Check sheet for the modelled part. Datum: model origin and axes. Units: mm. A direction names the side the tool comes from. Round coordinates to 2 decimals unless told otherwise and drop trailing zeros. Order: outer loops, then holes, each group sorted by start corner. A loop starts at its lowest first (then second) coordinate and runs counter-clockwise, first axis right, second up. Notation, with made-up numbers: (40.25, -4) -> (53.25, -4) arc R22 cw to (53.25, 4) -> close; hole circle Ø2 at (-14.5, 58.25). An arc over 180 degrees is marked (long way). Answer in a Markdown table with one row per item. Add a question column.
1. Sectioned sample at B-B, the plane z = 0. Record the boundary of the cut face in (x, y).
2. Sectioned sample at A-A, the plane x = 0. Record the boundary of the cut face in (y, z), then the cut area to 3 significant figures.
3. Depth check by flat-ended pin: P1, Ø1, axis at x = 5.5, y = 13, coming from the -Z side; P2, Ø1.5, axis at x = 2.5, y = -65.5, coming from the +Z side; P3, Ø1.5, axis at x = -5.5, z = 5.5, coming from the -Y side. Enter the tip coordinate at first touch or a pass-through.
4. Access from +Z, -Z, +X, -X, +Y, -Y to the whole of each face (thin tool, end or side, straight path). Record for faces 1 (the flat face through (-6, -24.5, -3)), 2 (the cylindrical face through (-5.158, -65.845, 3.955)), 3 (the flat face through (0, -105, 0)).
5. Material ranges on L1, parallel to Y at x = 0, z = -7; L2, parallel to Z at x = 3, y = 35; L3, parallel to Z at x = 2.25, y = -76.5, recorded low to high. Write a range as from..to.
6. Sectioned sample at C-C, the plane y = 29.5. Record the boundary of the cut face in (x, z).
Solid Edge part; units mm, degrees
sketch "Sketch1" plane through (0, 0, 0) normal (0, -1, 0) x (1, 0, 0)
  circle A0 centre (0, 0) radius 6.5
extrude "Protrusion1" add sketch "Sketch1" along normal mid plane 210
sketch "Sketch2" plane through (0, -28.5, 0) normal (0, -1, 0) x (0, 0, -1)
  circle A0 centre (0, 0) radius 9
extrude "ExtrudedProtrusion_2" add sketch "Sketch2" against normal blind 4
chamfer "Chamfer_1" distance 0.75 angle 45 1 edges at (-6.5, -105, 0)
properties part number "SMV-102-4" material "STEEL, 4140"
Answer key:
| question | item | result |
|---|---|---|
| 1 | outline | (-9, -28.5) -> (-6.5, -28.5) -> (-6.5, -104.25) -> (-5.75, -105) -> (5.75, -105) -> (6.5, -104.25) -> (6.5, -28.5) -> (9, -28.5) -> (9, -24.5) -> (6.5, -24.5) -> (6.5, 105) -> (-6.5, 105) -> (-6.5, -24.5) -> (-9, -24.5) -> close |
| 2 | outline | (-105, -5.75) -> (-104.25, -6.5) -> (-28.5, -6.5) -> (-28.5, -9) -> (-24.5, -9) -> (-24.5, -6.5) -> (105, -6.5) -> (105, 6.5) -> (-24.5, 6.5) -> (-24.5, 9) -> (-28.5, 9) -> (-28.5, 6.5) -> (-104.25, 6.5) -> (-105, 5.75) -> close |
| 2 | area | 2,750 mm² |
| 3 | P1 | stops at z = -4.15 |
| 3 | P2 | stops at z = 6.26 |
| 3 | P3 | stops at y = -28.5 |
| 4 | face 1 | +Y |
| 4 | face 2 | -Y |
| 4 | face 3 | +Z, -Z, +X, -X, -Y |
| 5 | L1 | y = -28.5..-24.5 |
| 5 | L2 | z = -5.77..5.77 |
| 5 | L3 | z = -6.1..6.1 |
| 6 | outline | circle Ø13 at (0, 0) |
